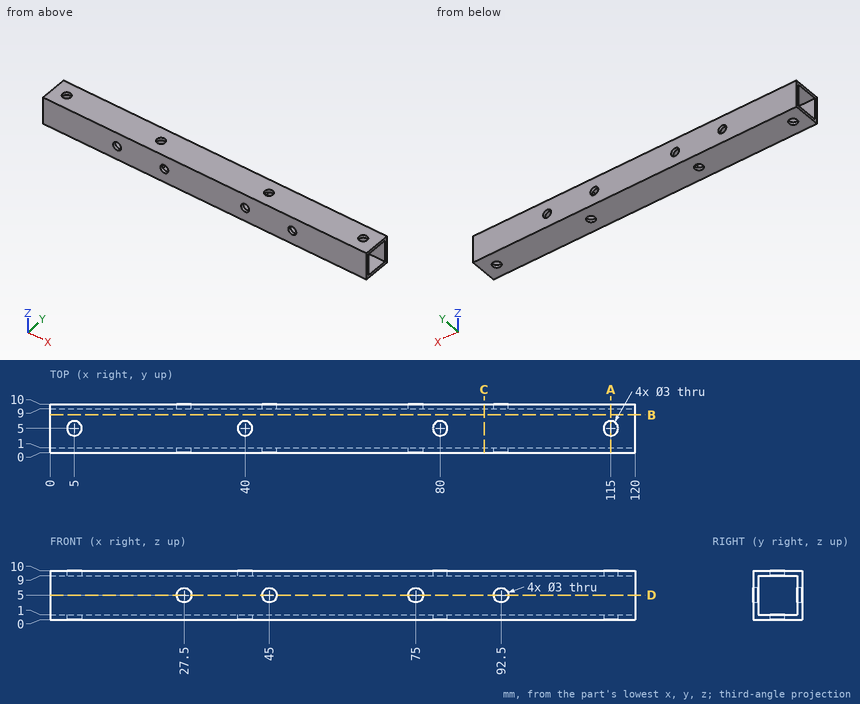
Check sheet for the drawn part. Datum: minimum x, y, z corner. Units: mm. Round coordinates to 2 decimals unless told otherwise and drop trailing zeros. Loops run counter-clockwise (first coordinate to the right, second up) from the corner with the lowest first, then second, coordinate; pieces in that order, holes last.
Item 1: Cross-section at C-C on x = 89. Record the boundary of the cut face in (y, z), then the cut area to 3 significant figures.
Item 2: Cross-section at B-B on y = 7.75. Record the boundary of the cut face in (x, z).
Item 3: Thickness scan on line 1 (X direction, y = 0.7, z = 5); line 2 (Z direction, x = 55, y = 5.25). Record the ranges inside material, lowest first.
Item 4: Gauge pin test, flat end, axial feed: pin 1 (1.8 mm diameter, centred on x = 40, y = 5, fed in from -Z). Record the tip position at first contact, or that the pin passes through.
Item 5: Cross-section at D-D on z = 5. Count the separate pieces of the cut face and the enclosed holes in it, then the cut area to 3 significant figures.
Item 6: Cross-section at A-A on x = 115. Record the boundary of the cut face in (y, z), then the cut area to 3 significant figures.
Answer sheet:
1. outline: (0, 0) - (10, 0) - (10, 10) - (0, 10) - close; hole (1, 1) - (9, 1) - (9, 9) - (1, 9) - close
1. area: 36.0 mm2
2. outline: (0, 0) - (120, 0) - (120, 1) - (0, 1) - close; (0, 9) - (120, 9) - (120, 10) - (0, 10) - close
3. line 1: x = 0 to 26, 29 to 43.5, 46.5 to 73.5, 76.5 to 91, 94 to 120
3. line 2: z = 0 to 1, 9 to 10
4. pin 1: passes through
5. separate pieces: 10
5. enclosed holes: 0
5. area: 216 mm2
6. outline: (0, 0) - (3.5, 0) - (3.5, 1) - (1, 1) - (1, 9) - (3.5, 9) - (3.5, 10) - (0, 10) - close; (6.5, 0) - (10, 0) - (10, 10) - (6.5, 10) - (6.5, 9) - (9, 9) - (9, 1) - (6.5, 1) - close
6. area: 30.0 mm2
